CAD build for the part. Positions are in the model's coordinates, mm. A direction names the side the tool comes from. Give positions to 0.01 mm unless a question says otherwise; leave off trailing zeros. Write each loop counter-clockwise with the first axis right and the second up, starting at its lowest first coordinate (ties: lowest second). Pieces come first, ordered by that corner, then holes. Notation, with made-up numbers: (-22, -17) - (-6, -17) arc R24 cw to (-6, 9) - close; hole circle Ø9 at (-14, 85). An arc over 180 degrees is marked (long way). Answer as a JSON object with one key per item and string values.
from build123d import *

# Parameters (mm, degrees)
SKETCH1_R           = 20
BOSS_EXTRUDE1_DEPTH = 1.5


with BuildPart() as part:
    # Sketch1 → Boss-Extrude1 (new body)
    with BuildSketch(Plane(origin=(0, 0, 0), x_dir=(1, 0, 0), z_dir=(0, 1, 0))):
        Circle(SKETCH1_R)
        with BuildLine():
            Line((11.03460466, 1.6), (12.95, 1.6))
            Line((12.95, 1.6), (12.95, -1.6))
            Line((12.95, -1.6), (11.03460466, -1.6))
            ThreePointArc((11.03460466, -1.6), (-11.15, 0), (11.03460466, 1.6))
        make_face(mode=Mode.SUBTRACT)
    extrude(amount=BOSS_EXTRUDE1_DEPTH)


solid = part.part
(1) Saw through at B-B, the plane y = 1.25. Give the cut face in (x, z), and give its area (3 significant figures).
Answer key:
{"outline": "circle Ø40 at (0, 0); hole (11.03, -1.6) - (12.95, -1.6) - (12.95, 1.6) - (11.03, 1.6) arc R11.15 ccw (long way) to start", "area": "860 mm²"}
(2) Saw through at C-C, the plane x = 0. Give the cut face in (y, z).
Answer key:
{"outline": "(0, -20) - (1.5, -20) - (1.5, -11.15) - (0, -11.15) - close; (0, 11.15) - (1.5, 11.15) - (1.5, 20) - (0, 20) - close"}
(3) Saw through at A-A, the plane z = 0. Give the cut face in (x, y), and give its area (4 significant figures).
Answer key:
{"outline": "(-20, 0) - (-11.15, 0) - (-11.15, 1.5) - (-20, 1.5) - close; (12.95, 0) - (20, 0) - (20, 1.5) - (12.95, 1.5) - close", "area": "23.85 mm²"}
(4) Pull direction Z, two halves, no side cores. Call faces 3 (the face through (12, 1, 1.6)), 4 (the face through (12.95, 1, 0)), 5 (the face through (-4.336, 0.74, 19.524)), 6 (the face through (9, 0, 9)): pulls with the +Z half, pulls with the -Z half, needs draft (parallel to the pull), parting line crosses it, or undercut.
Answer key:
{"face 3": "undercut", "face 4": "undercut", "face 5": "parting line crosses it", "face 6": "needs draft"}
(5) 3-axis set-ups, long thin cutter, end or side, ignore diameter. For faces 1 (the face through (12, 1, -1.6)), 2 (the face through (9, 1.5, 9)): which of +Z, -Z, +X, -X, +Y, -Y reach the whole face in a straight line?
Answer key:
{"face 1": "+Y, -Y", "face 2": "+Z, -Z, +X, -X, +Y"}
(6) Saw through at D-D, the plane z = 16.5. Give the cut face in (x, y), and give its area (3 significant figures).
Answer key:
{"outline": "(-11.3, 0) - (11.3, 0) - (11.3, 1.5) - (-11.3, 1.5) - close", "area": "33.9 mm²"}
(7) Probe L1, parallel to Z at x = 0, y = 0.8; L2, parallel to X at y = 1.2, z = 0; L3, parallel to X at y = 0.35, z = 10. List the from-to ranges inside material, lowest first. Write a range as [from, to].
Answer key:
{"L1": "z = [-20, -11.15], [11.15, 20]", "L2": "x = [-20, -11.15], [12.95, 20]", "L3": "x = [-17.32, -4.93], [4.93, 17.32]"}
